```python
from build123d import *

# Parameters (mm, degrees)
FILLET1_R          = 0.5
FILLET2_R          = 2
FILLET3_R          = 0.2
SKETCH3_R          = 6
CUT_EXTRUDE1_DEPTH = 0.1
SKETCH4_R          = 7.5
SKETCH4_R_2        = 3.1
CUT_EXTRUDE2_DEPTH = 0.1


with BuildPart() as part:
    # Sketch2 → Revolve1 (revolve)
    with BuildSketch(Plane(origin=(0, 0, 0), x_dir=(0, 0, -1), z_dir=(1, 0, 0)), mode=Mode.PRIVATE) as revolve1_sk:
        with BuildLine():
            Line((0, 0), (0, 9))
            Line((0, 9), (59.875, 9))
            ThreePointArc((59.875, 9), (60.5, 8.375), (61.125, 9))
            Line((61.125, 9), (64, 9))
            Line((64, 9), (64, 3.075))
            Line((64, 3.075), (65, 3.075))
            Line((65, 3.075), (65, 0))
            Line((65, 0), (0, 0))
        make_face()
    revolve(revolve1_sk.sketch.rotate(Axis((0, 0, 1000), (0, 0, -1)), 90), axis=Axis((0, 0, 1000), (0, 0, -1)))

    # Fillet1
    fillet1_edges = [part.edges().sort_by_distance(p)[0] for p in [
        (-9, 0, 0),
        (-9, 0, -64),
    ]]
    fillet(fillet1_edges, radius=FILLET1_R)

    # Fillet2
    fillet2_edges = [part.edges().sort_by_distance(p)[0] for p in [
        (-9, 0, -59.875),
        (-9, 0, -61.125),
    ]]
    fillet(fillet2_edges, radius=FILLET2_R)

    # Fillet3
    fillet3_edges = [part.edges().sort_by_distance(p)[0] for p in [
        (-3.075, 0, -65),
    ]]
    fillet(fillet3_edges, radius=FILLET3_R)

    # Sketch3 → Cut-Extrude1 (cut)
    with BuildSketch(Plane.XY):
        Circle(SKETCH3_R)
    extrude(amount=-CUT_EXTRUDE1_DEPTH, mode=Mode.SUBTRACT)

    # Sketch4 → Cut-Extrude2 (cut)
    with BuildSketch(Plane(origin=(0, 0, -64), x_dir=(-1, 0, 0), z_dir=(0, 0, -1))):
        Circle(SKETCH4_R)
        Circle(SKETCH4_R_2, mode=Mode.SUBTRACT)
    extrude(amount=-CUT_EXTRUDE2_DEPTH, mode=Mode.SUBTRACT)


solid = part.part
```
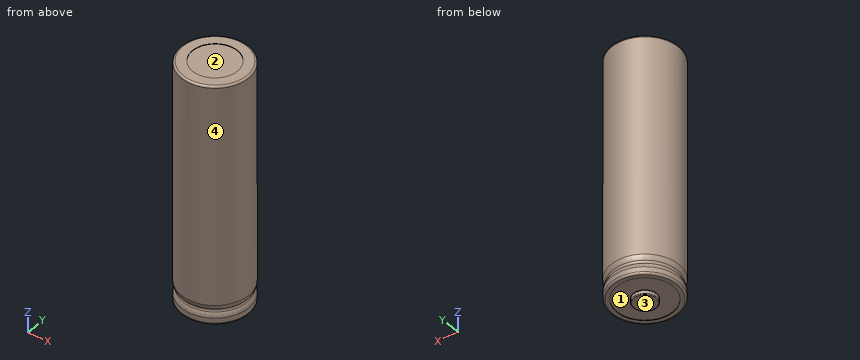
Work out the finished part from the listing and answer in its coordinate system (mm). Face numbers are marked on the shaded views. Give positions to 0.01 mm unless a question says otherwise; leave off trailing zeros. Write each loop counter-clockwise with the first axis right and the second up, starting at its lowest first coordinate (ties: lowest second). Pieces come first, ordered by that corner, then holes. Notation, with made-up numbers: (32.25, 65.5) -> (75.25, 65.5) arc R31 ccw to (75.25, 101.5) -> close; hole circle Ø1 at (0.5, 53.25). An arc over 180 degrees is marked (long way). Write item = value, one per line.
Q1. For a pull along X with two mould halves and no side action, classify the marked faces 1, 2, 3 and 4 as pulls with the +X half, pulls with the -X half, needs draft (parallel to the pull), parting line crosses it, or undercut.
Computed values:
face_1 = undercut
face_2 = undercut
face_3 = needs draft
face_4 = parting line crosses it
Q2. Consider line 1 along Z through (x, y) = (-6.75, 1.5); line 2 along Z through (x, y) = (-2.75, -3.25); line 3 along X through (y, z) = (-1.5, -20). Determine where each line is inside the solid, lowest interval first.
Computed values:
line_1 = -63.9 to 0
line_2 = -63.9 to -0.1
line_3 = -8.87 to 8.87
Q3. Flat-ended cylindrical pins translate along their axes: pin 1 Ø1.5 at (x, z) = (-6.5, -41.5) entering from +Y; pin 2 Ø1.5 at (x, y) = (4.5, 4) entering from -Z; pin 3 Ø4 at (x, y) = (2, -5.5) entering from +Z; pin 4 Ø2 at (y, z) = (3.5, -45) entering from -X. Find the tip coordinate at first contact, or state that the pin passes through.
Computed values:
pin_1 = 6.92
pin_2 = -63.9
pin_3 = 0
pin_4 = -8.65
Q4. Section A-A on z = -21.5 is taken. Determine the outline of the cut face in (x, y).
Computed values:
outline = circle Ø18 at (0, 0)
